Source: three-view drawing plus pictorial views. Frame: mm from the lowest corner of the part. Give positions to 0.01 mm unless a question says otherwise; leave off trailing zeros. Order: outer loops, then holes, each group sorted by start corner. A loop starts at its lowest first (then second) coordinate and runs counter-clockwise, first axis right, second up.
1) Section C-C, the plane y = 2.75. Give the number of separate pieces and of enclosed holes in the cut face, plus the area to 3 significant figures.
2) Section A-A, the plane z = 82.5. Return loops of the section in (x, y).
3) Section D-D, the plane z = 25. Return loops of the section in (x, y).
4) Material intervals for line 1 (Z direction, x = 75, y = 7.75); line 2 (X direction, y = 1.25, z = 78); line 3 (Z direction, x = 162, y = 7.75), sorted ascending.
5) First-contact query: P1, Ø5, axis at y = 3, z = 82.5, coming from the -X side. Flat tip, straight axial feed; report the tip coordinate or a pass-through.
6) Section B-B, the plane x = 25. Return loops of the section in (y, z).
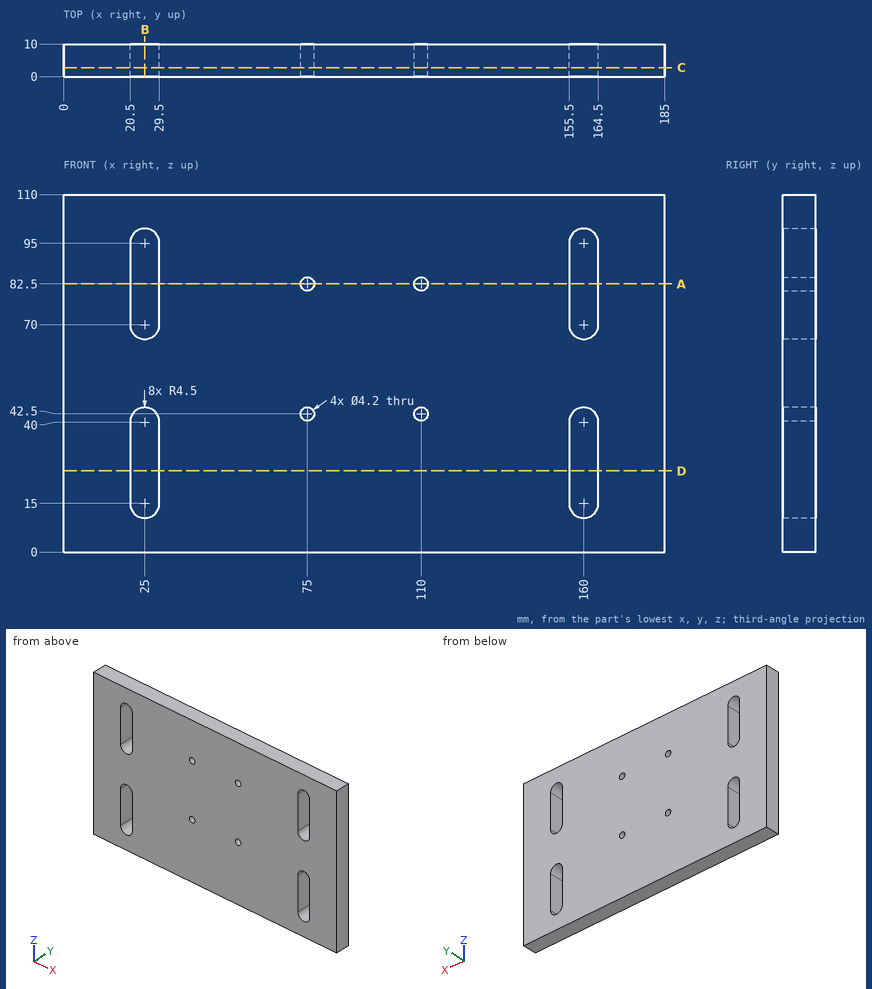
From the geometry:
1. separate pieces: 1
1. enclosed holes: 8
1. area: 19,100 mm2
2. outline: (0, 0) - (20.5, 0) - (20.5, 10) - (0, 10) - close; (29.5, 0) - (72.9, 0) - (72.9, 10) - (29.5, 10) - close; (77.1, 0) - (107.9, 0) - (107.9, 10) - (77.1, 10) - close; (112.1, 0) - (155.5, 0) - (155.5, 10) - (112.1, 10) - close; (164.5, 0) - (185, 0) - (185, 10) - (164.5, 10) - close
3. outline: (0, 0) - (20.5, 0) - (20.5, 10) - (0, 10) - close; (29.5, 0) - (155.5, 0) - (155.5, 10) - (29.5, 10) - close; (164.5, 0) - (185, 0) - (185, 10) - (164.5, 10) - close
4. line 1: z = 0 to 40.4, 44.6 to 80.4, 84.6 to 110
4. line 2: x = 0 to 20.5, 29.5 to 155.5, 164.5 to 185
4. line 3: z = 0 to 10.97, 44.03 to 65.97, 99.03 to 110
5. P1: stops at x = 0
6. outline: (0, 0) - (10, 0) - (10, 10.5) - (0, 10.5) - close; (0, 44.5) - (10, 44.5) - (10, 65.5) - (0, 65.5) - close; (0, 99.5) - (10, 99.5) - (10, 110) - (0, 110) - close
